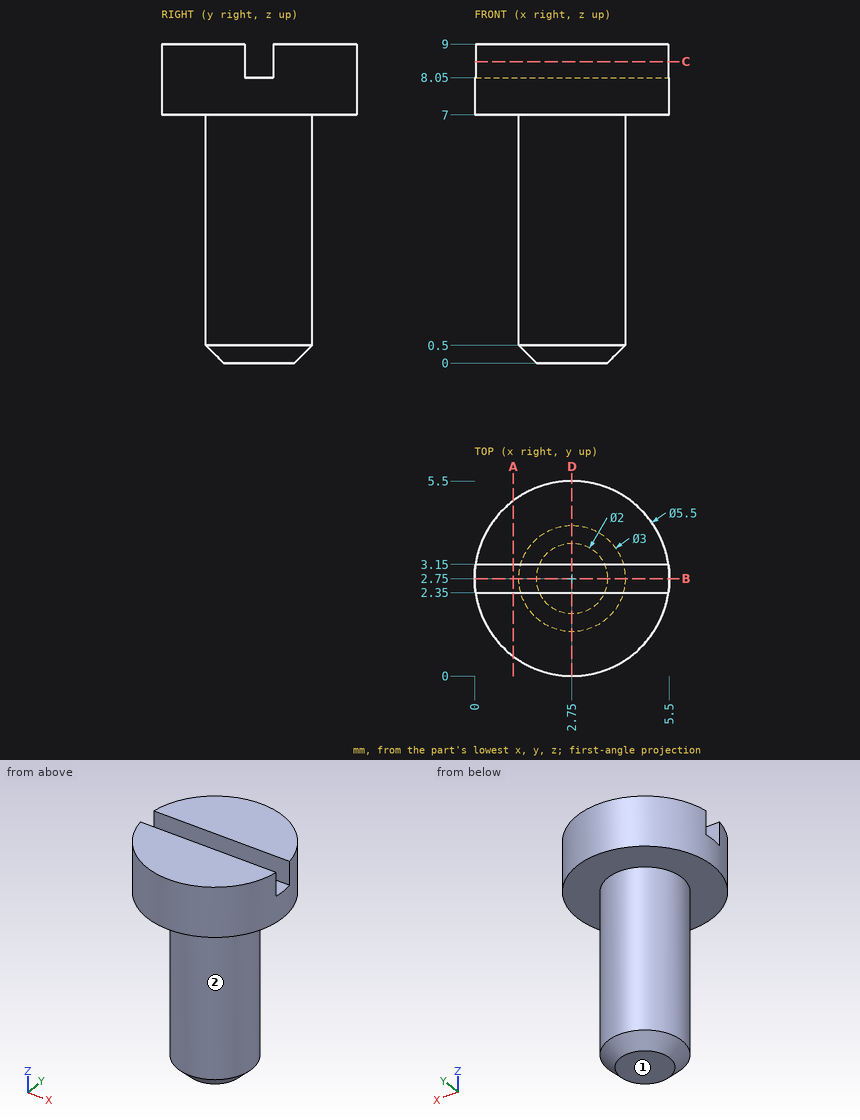
Input: dimensioned drawing with shaded views. Units: mm. Origin: part minimum x, y, z. A direction names the side the tool comes from. Give positions to 0.01 mm unless a question says otherwise; leave off trailing zeros. Write each loop counter-clockwise with the first axis right and the second up, starting at its lowest first coordinate (ties: lowest second). Pieces come first, ordered by that corner, then holes. Notation, with made-up numbers: M 24.25,82 L 42.25,82 A14 cw 42.25,94 Z; hole C -39.5,70.5 d11. An arc over 180 degrees is marked long. Write item = value, one per line. Start each with the question number.
1) Cut plane B-B on y = 2.75. Return the cut outline in (x, z), then the cut area to 3 significant figures.
2) Reachability of the marked faces 1 and 2 from +Z, -Z, +X, -X, +Y, -Y: full face, straight path, thin tool, end or side. Return the list, or none.
3) Cut plane C-C on z = 8.5. Return the cut outline in (x, y), then the cut area to 3 significant figures.
4) Cut plane A-A on x = 1.1. Return the cut outline in (y, z).
5) Material intervals for line 1 along Z through (x, y) = (4.5, 4.65); line 2 along Z through (x, y) = (2.25, 2.5); line 3 along Y through (x, z) = (1.55, 8.75), sorted ascending. Write a range as [from, to].
6) Cut plane D-D on x = 2.75. Return the cut outline in (y, z), then the cut area to 3 significant figures.
7) First-contact query: pin 1 Ø1 at (x, z) = (2, 8.5) entering from -Y; pin 2 Ø0.8 at (x, z) = (1.5, 8.5) entering from +Y; pin 3 Ø3 at (y, z) = (1.5, 3) entering from -X. Flat tips, straight axial feed; report the tip coordinate or a pass-through.
Solved:
q1.outline = M 0,7 L 1.25,7 L 1.25,0.5 L 1.75,0 L 3.75,0 L 4.25,0.5 L 4.25,7 L 5.5,7 L 5.5,8.05 L 0,8.05 Z
q1.area = 26.5 mm2
q2.face_1 = -Z, +X, -X, +Y, -Y
q2.face_2 = -Z
q3.outline = M 0.03,2.35 A2.75 ccw 5.47,2.35 Z; M 0.03,3.15 L 5.47,3.15 A2.75 ccw Z
q3.area = 19.4 mm2
q4.outline = M 0.55,7 L 4.95,7 L 4.95,9 L 3.15,9 L 3.15,8.05 L 2.35,8.05 L 2.35,9 L 0.55,9 Z
q5.line_1 = [7, 9]
q5.line_2 = [0, 8.05]
q5.line_3 = [0.28, 2.35], [3.15, 5.22]
q6.outline = M 0,7 L 1.25,7 L 1.25,0.5 L 1.75,0 L 3.75,0 L 4.25,0.5 L 4.25,7 L 5.5,7 L 5.5,9 L 3.15,9 L 3.15,8.05 L 2.35,8.05 L 2.35,9 L 0,9 Z
q6.area = 31.0 mm2
q7.pin_1 = 0.01
q7.pin_2 = 5.37
q7.pin_3 = 1.25
